```python
from build123d import *

# Parameters (mm, degrees)
BOX003_W                  = 100
BOX003_H                  = 10
BOX003_DEPTH              = 25
SKETCH003_W               = 90.806315
SKETCH003_H               = 20.169361
POCKET_DEPTH              = 10.001
BOX005_W                  = 100
BOX005_H                  = 10
BOX005_DEPTH              = 60
SKETCH004_W               = 91.218086
SKETCH004_H               = 40.361668
POCKET001_DEPTH           = 10.001
SKETCH005_W               = 70.455691
SKETCH005_H               = 22.66835
POCKET002_DEPTH           = 5
BOX004_W                  = 100
BOX004_H                  = 10
BOX004_DEPTH              = 10
BOX001_W                  = 65
BOX001_H                  = 20
BOX001_DEPTH              = 20
ARRAY001_Y_COUNT          = 3
ARRAY001_Y_PITCH          = 58
BOX_W                     = 65
BOX_H                     = 20
BOX_DEPTH                 = 20
ARRAY_Y_COUNT             = 3
ARRAY_Y_PITCH             = 57
SKETCH_W                  = 19.999652
SKETCH_H                  = 20.000471
FUSION002_ROLL_ANGLE      = -0.066054
FUSION002_PITCH_ANGLE     = -0.217392
FUSION002_PLACEMENT_ANGLE = -0.581856
BOX002_W                  = 100
BOX002_H                  = 10
BOX002_DEPTH              = 10
BOX006_W                  = 20
BOX006_H                  = 20
BOX006_DEPTH              = 35
ARRAY002_X_COUNT          = 2
ARRAY002_X_PITCH          = 80
BOX007_W                  = 100
BOX007_H                  = 135
BOX007_DEPTH              = 2
FILLET008_R               = 1
FILLET009_R               = 1
SKETCH006_W               = 83.27878
SKETCH006_H               = 48.60762
POCKET003_DEPTH           = 2


with BuildPart() as pocket:
    # Box003 → Box003 (new body)
    with BuildSketch(Plane(origin=(-10, 35, 60), x_dir=(1, 0, 0), z_dir=(0, 0, 1))):
        with Locations((50, 5)):
            Rectangle(BOX003_W, BOX003_H)
    extrude(amount=BOX003_DEPTH)

    # Sketch003 → Pocket (cut, through all)
    with BuildSketch(Plane(origin=(-10, 35, 60), x_dir=(1, 0, 0), z_dir=(0, -1, 0))):
        with Locations((50.00284, 9.885892)):
            Rectangle(SKETCH003_W, SKETCH003_H)
    extrude(amount=-POCKET_DEPTH, mode=Mode.SUBTRACT)


with BuildPart() as pocket002:
    # Box005 → Box005 (new body)
    with BuildSketch(Plane(origin=(-9, 100, 60), x_dir=(1, 0, 0), z_dir=(0, 0, 1))):
        with Locations((50, 5)):
            Rectangle(BOX005_W, BOX005_H)
    extrude(amount=BOX005_DEPTH)

    # Sketch004 → Pocket001 (cut, through all)
    with BuildSketch(Plane(origin=(-9, 100, 60), x_dir=(1, 0, 0), z_dir=(0, -1, 0))):
        with Locations((49.065182, 20.377592)):
            Rectangle(SKETCH004_W, SKETCH004_H)
    extrude(amount=-POCKET001_DEPTH, mode=Mode.SUBTRACT)

    # Sketch005 → Pocket002 (cut)
    with BuildSketch(Plane(origin=(-9, 110, 60), x_dir=(-1, 0, 0), z_dir=(0, 1, 0))):
        with Locations((-48.841116, 49.679405)):
            Rectangle(SKETCH005_W, SKETCH005_H)
    extrude(amount=-POCKET002_DEPTH, mode=Mode.SUBTRACT)


with BuildPart() as obj1:
    # Box004 → Box004 (new body)
    with BuildSketch(Plane(origin=(-9, 125, 60), x_dir=(1, 0, 0), z_dir=(0, 0, 1))):
        with Locations((50, 5)):
            Rectangle(BOX004_W, BOX004_H)
    extrude(amount=BOX004_DEPTH)


with BuildPart() as obj2:
    # Box001 → Box001 (new body)
    with BuildSketch(Plane(origin=(7, 0, 40), x_dir=(1, 0, 0), z_dir=(0, 0, 1))):
        with Locations((32.5, 10)):
            Rectangle(BOX001_W, BOX001_H)
    extrude(amount=BOX001_DEPTH)

    # Array001 Y: obj2 ×3


with BuildPart() as obj2_1:
    add(obj2.part)
    with Locations(*[(0, i * ARRAY001_Y_PITCH, 0) for i in range(1, ARRAY001_Y_COUNT)]):
        add(obj2.part)


with BuildPart() as obj3:
    # Box → Box (new body)
    with BuildSketch(Plane(origin=(7, 0, -10), x_dir=(1, 0, 0), z_dir=(0, 0, 1))):
        with Locations((32.5, 10)):
            Rectangle(BOX_W, BOX_H)
    extrude(amount=BOX_DEPTH)

    # Array Y: obj3 ×3


with BuildPart() as obj3_1:
    add(obj3.part)
    with Locations(*[(0, i * ARRAY_Y_PITCH, 0) for i in range(1, ARRAY_Y_COUNT)]):
        add(obj3.part)


with BuildPart() as obj4:
    # Sweep: sweep along a path in Sketch001
    with BuildLine(Plane.YZ) as sweep_path:
        Line((0, 0), (133.575411, -0.011573))
        ThreePointArc((133.575411, -0.011573), (145.205679, 4.807053), (150.018155, 16.439868))
        Line((150.018155, 16.439868), (150.005868, 36.408139))
        ThreePointArc((150.005868, 36.408139), (146.034392, 45.985141), (136.455834, 49.952864))
        Line((136.455834, 49.952864), (0, 49.98336))
    # Sketch → Sweep (sweep)
    with BuildSketch(Plane.XZ):
        with Locations((0.000263, -0.000434)):
            Rectangle(SKETCH_W, SKETCH_H)
    sweep(path=sweep_path.line)


with BuildPart() as obj5:
    # Fusion base: copy of obj4
    add(obj4.part)

    # Fusion: union obj3
    add(obj3_1.part)


with BuildPart() as obj6:
    # Part__Mirroring: instance of obj4
    add(obj4.part.mirror(Plane(origin=(0, 0, 0), x_dir=(0, -1, 0), z_dir=(1, 0, 0))))


with BuildPart() as obj6_1:
    # Part__Mirroring placement: moved
    add(obj6.part.moved(Location((80, 0, 0))))

    # Fusion001: union obj5
    add(obj5.part)

    # Fusion002: union obj2
    add(obj2_1.part)


with BuildPart() as obj6_2:
    # Fusion002 roll: moved
    add(obj6_1.part.rotate(Axis((0, 0, 0), (1, 0, 0)), FUSION002_ROLL_ANGLE))


with BuildPart() as obj6_3:
    # Fusion002 pitch: moved
    add(obj6_2.part.rotate(Axis((0, 0, 0), (0, 1, 0)), FUSION002_PITCH_ANGLE))


with BuildPart() as obj6_4:
    # Fusion002 placement: moved
    add(obj6_3.part.moved(Location((-0.067416, 0.088109, 0.519024))).rotate(Axis((-0.067416, 0.088109, 0.519024), (0, 0, 1)), FUSION002_PLACEMENT_ANGLE))


with BuildPart() as obj7:
    # Box002 → Box002 (new body)
    with BuildSketch(Plane(origin=(-10, 0, 60), x_dir=(1, 0, 0), z_dir=(0, 0, 1))):
        with Locations((50, 5)):
            Rectangle(BOX002_W, BOX002_H)
    extrude(amount=BOX002_DEPTH)

    # Fusion003: union obj6
    add(obj6_4.part)


with BuildPart() as fusion004:
    # Box006 → Box006 (new body)
    with BuildSketch(Plane(origin=(-10, 0, 8), x_dir=(1, 0, 0), z_dir=(0, 0, 1))):
        with Locations((10, 10)):
            Rectangle(BOX006_W, BOX006_H)
    extrude(amount=BOX006_DEPTH)

    # Array002 X: Fusion004 ×2


with BuildPart() as fusion004_1:
    add(fusion004.part)
    with Locations(*[(i * ARRAY002_X_PITCH, 0, 0) for i in range(1, ARRAY002_X_COUNT)]):
        add(fusion004.part)

    # Fusion004: union obj7
    add(obj7.part)


with BuildPart() as pocket003:
    # Box007 → Box007 (new body)
    with BuildSketch(Plane(origin=(-10, 0, -11), x_dir=(1, 0, 0), z_dir=(0, 0, 1))):
        with Locations((50, 67.5)):
            Rectangle(BOX007_W, BOX007_H)
    extrude(amount=BOX007_DEPTH)

    # Fusion005: union Fusion004
    add(fusion004_1.part)

    # Fusion006: union Pocket, Pocket002, obj1
    add(pocket.part)
    add(pocket002.part)
    add(obj1.part)

    # Fillet008
    fillet008_edges = [pocket003.edges().sort_by_distance(p)[0] for p in [
        (41, 135, 70),
        (41, 125, 70),
        (40, 45, 85),
        (40, 35, 85),
    ]]
    fillet(fillet008_edges, radius=FILLET008_R)

    # Fillet009
    fillet009_edges = [pocket003.edges().sort_by_distance(p)[0] for p in [
        (40, 10, 70),
        (-2.193365, 110, 120),
        (41, 100, 120),
        (40, 0, 70),
        (83.034481, 110, 120),
        (39.841116, 105, 120),
    ]]
    fillet(fillet009_edges, radius=FILLET009_R)

    # Sketch006 → Pocket003 (cut)
    with BuildSketch(Plane.XY.offset(60.196758)):
        with Locations((46.096251, 113.947426)):
            Rectangle(SKETCH006_W, SKETCH006_H)
    extrude(amount=-POCKET003_DEPTH, mode=Mode.SUBTRACT)


solid = pocket003.part
```
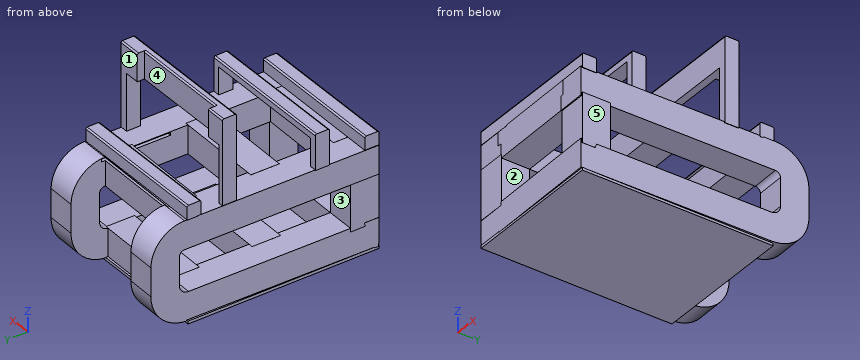
Here's how the part is built. I have some questions about the finished solid (model axes, mm). Face numbers are marked on the shaded views. A direction names the side the tool comes from. Coordinates: 2 decimals unless noted, no trailing zeros. Order: outer loops, then holes, each group sorted by start corner. A loop starts at its lowest first (then second) coordinate and runs counter-clockwise, first axis right, second up.
1) Imagine slicing it at D-D on y = 122. State how many separate pieces and enclosed holes the cut face has, and give its area (3 significant figures).
2) I need wall thicknesses on line 1 (Z direction, x = 87.5, y = 109); line 2 (Z direction, x = 73.5, y = 42.5); line 3 (Z direction, x = 81.5, y = 87.5). Which ranges of each line are inside material? Lowest first, please.
3) Imagine slicing it at C-C on z = 33.5. List the corners of the cut face in (x, y) for me, and give its area (3 significant figures).
4) We'd pull the mould along Y, two halves only. Please class the marked faces 3, 4 and 5: +Y half, -Y half, draft (parallel to the pull), parting line (faces both ways), or undercut.
5) Which directions (+Z, -Z, +X, -X, +Y, -Y) give clear straight access to the entire face, cutting with the end or side of a thin tool? Please do the marked faces 1 and 2.
6) Imagine slicing it at A-A on y = 85.5. List the corners of the cut face in (x, z) for me.
7) Will these pins go through, and if not, where does the flat tip stop? pin 1 (2 mm diameter, centred on x = 5, z = 82.5, fed in from -Y); pin 2 (11.5 mm diameter, centred on x = 35.5, y = 35.5, fed in from +Z); pin 3 (6 mm diameter, centred on y = 9.5, z = 27.5, fed in from +X).
Response values:
1. separate pieces: 2
1. enclosed holes: 1
1. area: 3,990 mm2
2. line 1: z = -11 to 10.71, 40.68 to 58.2, 60.2 to 120
2. line 2: z = -11 to 10.74, 40.72 to 60.72, 79.97 to 85
2. line 3: z = -11 to 10.72, 40.69 to 60.69
3. outline: (-10, 0) - (10, 0) - (10, 20) - (-10, 20) - close; (-8.77, 140.23) - (11.23, 140.03) - (11.43, 160.03) - (-8.57, 160.23) - close; (70, 0) - (90, 0) - (90, 20) - (70, 20) - close; (71.23, 139.42) - (91.23, 139.21) - (91.43, 159.21) - (71.43, 159.42) - close
3. area: 1,600 mm2
4. face 3: undercut
4. face 4: +Y half
4. face 5: draft
5. face 1: +Z, +X, -X
5. face 2: -Y
6. outline: (-10, -11) - (90, -11) - (90, -9.25) - (90.84, -9.25) - (90.77, 10.75) - (70.77, 10.68) - (70.84, -9) - (10.84, -9) - (10.76, 10.45) - (-9.24, 10.38) - (-9.16, -9) - (-10, -9) - close; (-9.43, 60.35) - (-9.35, 40.35) - (10.65, 40.42) - (10.57, 60.42) - close; (70.58, 60.65) - (70.65, 40.65) - (90.65, 40.72) - (90.58, 60.73) - close
7. pin 1: stops at y = 35
7. pin 2: stops at z = 85
7. pin 3: stops at x = 90
